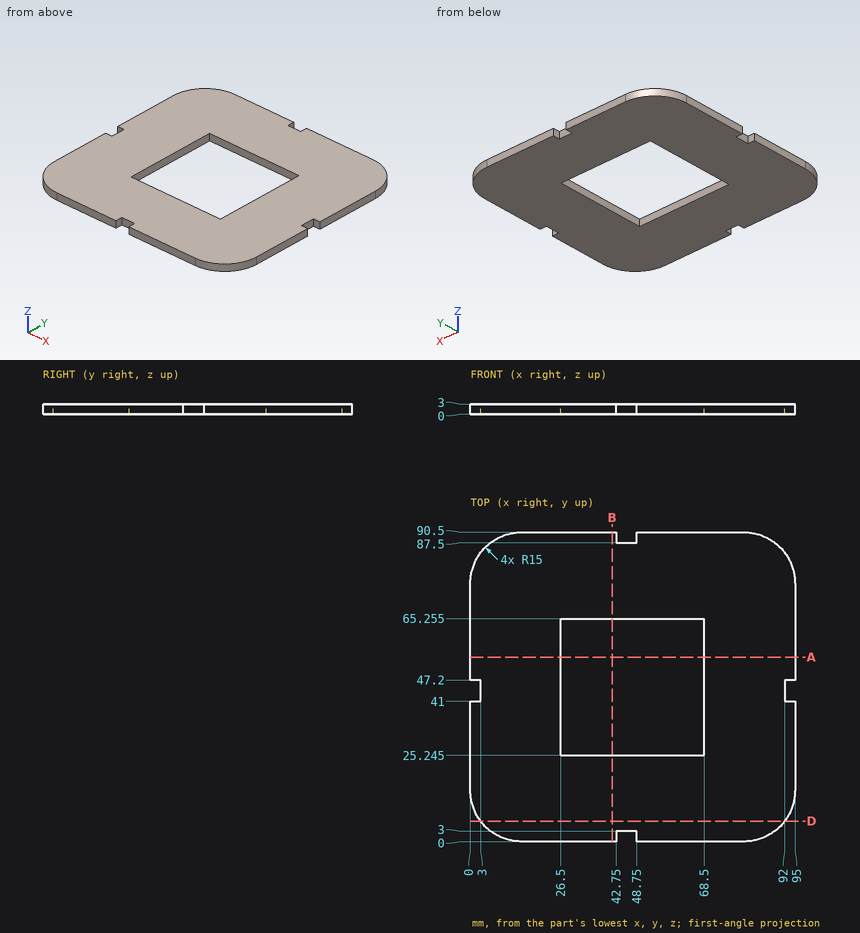
Source: three-view drawing plus pictorial views. Frame: mm from the lowest corner of the part. Round coordinates to 2 decimals unless told otherwise and drop trailing zeros. Loops run counter-clockwise (first coordinate to the right, second up) from the corner with the lowest first, then second, coordinate; pieces in that order, holes last.
Q1. Section D-D on y = 6. Return loops of the section in (x, z), plus the area to 3 significant figures.
Q2. Section B-B on x = 41.5. Return loops of the section in (y, z) (1 decimal).
Q3. Section A-A on y = 54. Return loops of the section in (x, z), plus the area to 3 significant figures.
Q4. Material intervals for L1, parallel to Y at x = 41, z = 0.9 (1 decimal); L2, parallel to X at y = 35, z = 1.75; L3, parallel to X at y = 42.5, z = 1.75, sorted ascending.
Q5. Pin query (flat end, axial travel): P1, Ø1.5, axis at y = 78.5, z = 2, coming from the +X side; P2, Ø1.5, axis at x = 94, z = 1.5, coming from the -Y side; P3, Ø1.5, axis at x = 94, z = 1, coming from the +Y side. Return the tip coordinate at first contact, or that it passes through.
Evaluation:
1. outline: (3, 0) - (92, 0) - (92, 3) - (3, 3) - close
1. area: 267 mm2
2. outline: (0, 0) - (25.2, 0) - (25.2, 3) - (0, 3) - close; (65.3, 0) - (90.5, 0) - (90.5, 3) - (65.3, 3) - close
3. outline: (0, 0) - (26.5, 0) - (26.5, 3) - (0, 3) - close; (68.5, 0) - (95, 0) - (95, 3) - (68.5, 3) - close
3. area: 159 mm2
4. L1: y = 0 to 25.2, 65.3 to 90.5
4. L2: x = 0 to 26.5, 68.5 to 95
4. L3: x = 3 to 26.5, 68.5 to 92
5. P1: stops at x = 94.83
5. P2: stops at y = 7.97
5. P3: stops at y = 82.53
